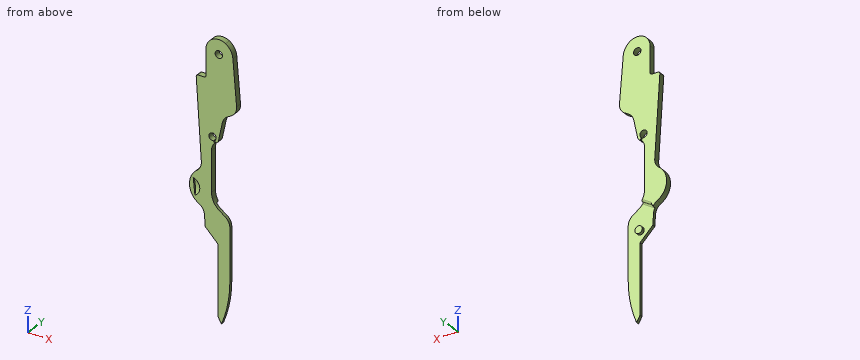
```python
from build123d import *

# Parameters (mm, degrees)
BOSS_EXTRUDE1_DEPTH     = 0.8
FILLET1_R               = 4.2
SKETCH2_R               = 1
CUT_EXTRUDE1_DEPTH      = 75.905340264
CUT_EXTRUDE2_DEPTH      = 75.905340264
CUT_EXTRUDE_THIN1_DEPTH = 75.905340264
FILLET2_R               = 3
CUT_EXTRUDE4_DEPTH      = 0.8
FILLET3_R               = 5
FILLET4_R               = 0.4
FILLET5_R               = 3
FILLET6_R               = 1
SKETCH6_R               = 1
BOSS_EXTRUDE2_DEPTH     = 0.8
SKETCH7_W               = 3
SKETCH7_H               = 11.1
CUT_EXTRUDE5_DEPTH      = 75.882809828
FILLET7_R               = 0.5
FILLET8_R               = 0.5
FILLET10_R              = 3.5
CUT_EXTRUDE6_DEPTH      = 0.5
FILLET11_R              = 2.4


# Some blends are built 0.0001 mm under size
with BuildPart() as part:
    # Sketch1 → Boss-Extrude1 (new, symmetric)
    with BuildSketch(Plane(origin=(0, 0, 0), x_dir=(1, 0, 0), z_dir=(0, 1, 0))):
        with BuildLine():
            Line((0, 0), (0, 6))
            Line((0, 6), (1.865312064, 35.32161706))
            ThreePointArc((1.865312064, 35.32161706), (-1.478238126, 40.437157563), (2.486591749, 45.087771133))
            Line((2.486591749, 45.087771133), (3.611473385, 62.770253978))
            ThreePointArc((3.611473385, 62.770253978), (4.720909281, 68.611088902), (7.232052008, 74))
            ThreePointArc((7.232052008, 74), (8.927699757, 68.307599169), (9.5, 62.395651864))
            Line((9.5, 62.395651864), (9.5, 46.645651864))
            Line((9.5, 46.645651864), (4.5, 43.144614173))
            Line((4.5, 43.144614173), (4.5, 27.994614173))
            Line((4.5, 27.994614173), (6.3, 26.955383689))
            Line((6.3, 26.955383689), (7.743698597, 20.163315799))
            Line((7.743698597, 20.163315799), (11.5, 17.994614173))
            Line((11.5, 17.994614173), (10, 0))
            Line((10, 0), (0, 0))
        make_face()
    extrude(amount=BOSS_EXTRUDE1_DEPTH, both=True)

    # Fillet1
    fillet1_edges = [part.edges().sort_by_distance(p)[0] for p in [
        (10, 0, 0),
    ]]
    fillet(fillet1_edges, radius=FILLET1_R)

    # Sketch2 → Cut-Extrude1 (cut, through all)
    with BuildSketch(Plane(origin=(0, 0.8, 0), x_dir=(1, 0, 0), z_dir=(0, 1, 0))):
        with Locations(Location((6.5, 4, 0), (0, 0, 270))):
            Circle(SKETCH2_R)
    extrude(amount=-CUT_EXTRUDE1_DEPTH, mode=Mode.SUBTRACT)

    # Sketch3 → Cut-Extrude2 (cut, through all)
    with BuildSketch(Plane(origin=(0, 0.8, 0), x_dir=(1, 0, 0), z_dir=(0, 1, 0))):
        with BuildLine():
            Line((5.640057539, 27.969251754), (5.047431638, 26.942793585))
            ThreePointArc((5.047431638, 26.942793585), (4.386066515, 25.063581102), (5.367538565, 26.797235046))
            Line((5.367538565, 26.797235046), (5.94316643, 27.794251754))
            Line((5.94316643, 27.794251754), (5.640057539, 27.969251754))
        make_face()
    extrude(amount=-CUT_EXTRUDE2_DEPTH, mode=Mode.SUBTRACT)

    # Sketch4 → Cut-Extrude-Thin1 (cut, through all)
    with BuildSketch(Plane(origin=(0, 0.8, 0), x_dir=(1, 0, 0), z_dir=(0, 1, 0))):
        Polygon((6.299086102, 72.375061168), (6.299086102, 53.5), (2.799086102, 50), (-4.271981709, 57.071067812), (-3.700913898, 57.642135624), (-3.700913898, 72.375061168), align=None)
    extrude(amount=-CUT_EXTRUDE_THIN1_DEPTH, mode=Mode.SUBTRACT)

    # Fillet2
    fillet2_edges = [part.edges().sort_by_distance(p)[0] for p in [
        (1.865312064, 0, -35.32161706),
        (2.486591749, 0, -45.087771133),
        (9.5, 0, -46.645651864),
    ]]
    fillet(fillet2_edges, radius=FILLET2_R)

    # Sketch5 → Cut-Extrude4 (cut)
    with BuildSketch(Plane(origin=(0, 0.8, 0), x_dir=(1, 0, 0), z_dir=(0, 1, 0))):
        Polygon((2.486591749, 45.087771133), (13.455116217, 38.22222401), (13.455116217, 80.886155846), (2.486591749, 80.886155846), (1.62289593, 47.027246142), align=None)
    extrude(amount=-CUT_EXTRUDE4_DEPTH, mode=Mode.SUBTRACT)

    # Fillet3
    fillet3_edges = [part.edges().sort_by_distance(p)[0] for p in [
        (4.5, 0, -43.144614173),
    ]]
    fillet(fillet3_edges, radius=FILLET3_R)

    # Fillet4
    fillet4_edges = [part.edges().sort_by_distance(p)[0] for p in [
        (3.91002639, 0, -44.196798274),
        (3.91002639, 0.8, -44.196798274),
    ]]
    fillet(fillet4_edges, radius=FILLET4_R - 0.0001)  # a hair under: the kernel refuses the full size

    # Fillet5
    # the kernel refuses this fillet: 3 mm, written as the material it adds along each edge
    with BuildSketch(Plane(origin=(4.5, 0.8, -27.994614173), x_dir=(0.8660254037844444, 0, 0.49999999999999023), z_dir=(0, -1, 0))) as fillet5_piece_1:
        with BuildLine():
            CenterArc((1.793781136, -2.893079935), FILLET5_R, 105.342812505, 44.657187495)
            Line((-0.804295075, -1.393079935), (0, 0))
            Line((0, 0), (1, 0))
        make_face()
    extrude(amount=1.6)
    with BuildSketch(Plane(origin=(7.743698597, 0.8, -20.163315799), x_dir=(0.8660254037844403, 0, 0.49999999999999734), z_dir=(0, -1, 0))) as fillet5_piece_2:
        with BuildLine():
            CenterArc((FILLET5_R * 0.445228685309, -FILLET5_R), FILLET5_R, 90, 48)
            Line((-FILLET5_R * 0.297916140169, -FILLET5_R * 0.330869393641), (0, 0))
            Line((0, 0), (FILLET5_R * 0.445228685309, 0))
        make_face()
    extrude(amount=1.6)
    # the kernel refuses this fillet: 3 mm, written as the material it takes off along each edge
    with BuildSketch(Plane(origin=(11.5, -5.55643762, -17.994614173), x_dir=(-0.86602540378444, 0, -0.49999999999999756), z_dir=(0, 1, 0))) as fillet5_2_piece_1:
        with BuildLine():
            CenterArc((FILLET5_R * 0.634191682642, FILLET5_R), FILLET5_R, 205.234939105, 64.765060895)
            Line((-FILLET5_R * 0.270375560362, FILLET5_R * 0.573669021903), (0, 0))
            Line((0, 0), (FILLET5_R * 0.634191682642, 0))
        make_face()
    extrude(amount=11.11287524, mode=Mode.SUBTRACT)

    # Fillet6
    fillet6_edges = [part.edges().sort_by_distance(p)[0] for p in [
        (6.3, 0, -26.955383689),
    ]]
    fillet(fillet6_edges, radius=FILLET6_R)

    # Sketch6 → Boss-Extrude2 (add)
    with BuildSketch(Plane(origin=(0, 0, 0), x_dir=(1, 0, 0), z_dir=(0, 1, 0))):
        with Locations(Location((6.14, 50.5, 0), (0, 0, 90))):
            Circle(SKETCH6_R)
    extrude(amount=BOSS_EXTRUDE2_DEPTH)

    # Sketch7 → Cut-Extrude5 (cut, through all)
    with BuildSketch(Plane(origin=(0, 0.8, 0), x_dir=(1, 0, 0), z_dir=(0, 1, 0))):
        with Locations((1.5, 5.55)):
            Rectangle(SKETCH7_W, SKETCH7_H)
    extrude(amount=-CUT_EXTRUDE5_DEPTH, mode=Mode.SUBTRACT)

    # Fillet7
    fillet7_edges = [part.edges().sort_by_distance(p)[0] for p in [
        (0.324439526, 0, -11.1),
    ]]
    fillet(fillet7_edges, radius=FILLET7_R)

    # Fillet8
    fillet8_edges = [part.edges().sort_by_distance(p)[0] for p in [
        (3, 0, -11.1),
    ]]
    fillet(fillet8_edges, radius=FILLET8_R)

    # Fillet10
    fillet10_edges = [part.edges().sort_by_distance(p)[0] for p in [
        (3, 0, 0),
    ]]
    fillet(fillet10_edges, radius=FILLET10_R)

    # Sketch8 → Cut-Extrude6 (cut)
    with BuildSketch(Plane.XZ.offset(0.8)):
        with BuildLine():
            Line((0, -42.705581243), (-0.472751816, -38.234175203))
            ThreePointArc((-0.472751816, -38.234175203), (1.308763911, -40.306514027), (0, -42.705581243))
        make_face()
    extrude(amount=-CUT_EXTRUDE6_DEPTH, mode=Mode.SUBTRACT)

    # Fillet11
    # the kernel refuses this fillet: 2.4 mm, written as the material it adds along each edge
    with BuildSketch(Plane(origin=(-1.081254443, -0.3, -40.559205352), x_dir=(-0.9553191525831795, 0, 0.2955762451682408), z_dir=(-0.2955762451682408, 0, -0.9553191525831795))) as fillet11_piece_1_section:
        with BuildLine():
            CenterArc((0.937051647, -2.4), FILLET11_R, 52.341537994, 37.658462006)
            Line((0.937051647, 0), (0.937051647, 0.048))
            Line((0.937051647, 0.048), (2.403339477, 0.048))
            Line((2.403339477, 0.048), (2.451339477, 0))
            ThreePointArc((2.451339477, 0), (2.451339477, -0.25), (2.432665233, -0.462))
            Line((2.432665233, -0.462), (2.403339477, -0.5))
        make_face()
    fillet11_piece_1 = revolve(axis=Axis((-1.081254443, -0.3, -40.559205352), (0, 1, 0)), revolution_arc=313.54514328, mode=Mode.PRIVATE)
    fillet11_piece_1 = split(fillet11_piece_1, bisect_by=Plane(origin=(-0.236375908, -0.3, -40.469878223), z_dir=(0.9944572448546122, 0, 0.1051417526778682)), keep=Keep.TOP, mode=Mode.PRIVATE)
    add(fillet11_piece_1)


solid = part.part
```
Build history of the part. All positions in model axes, mm. Round coordinates to 2 decimals unless told otherwise and drop trailing zeros. Write each loop counter-clockwise with the first axis right and the second up, starting at its lowest first coordinate (ties: lowest second). Pieces come first, ordered by that corner, then holes. Notation, with made-up numbers: (7.5, -40) - (16.5, -40) arc R28 ccw to (16.5, -8) - close; hole circle Ø1 at (88.25, -29.5). An arc over 180 degrees is marked (long way). Write each question's results on one line, items separated by ' | '. Start each with the question number.
Item 1: Saw through at A-A (z = -15). Write the cut outline in (x, y).
Item 2: Saw through at B-B (z = -37). Write the cut outline in (x, y), and give its area (3 significant figures).
Item 3: Wall check: L1, parallel to X at y = 0.55, z = -4; L2, parallel to Y at x = 5.25, z = -44; L3, parallel to Z at x = 6, y = 0.25. Give the ranges that are in metal, low to high. Write a range as [from, to].
Item 4: Drop flat-ended pins along their axis: P1, Ø6, axis at x = 7, z = -66.5, coming from the +Y side; P2, Ø0.9, axis at y = -0.5, z = -59, coming from the -X side; P3, Ø0.5, axis at y = 0.5, z = -6.5, coming from the -X side. Give the stop position or say it passes through.
Results are:
1) outline: (0.57, -0.8) - (11.25, -0.8) - (11.25, 0.8) - (0.57, 0.8) - close
2) outline: (-0.43, -0.8) - (4.5, -0.8) - (4.5, 0.8) - (-0.43, 0.8) - close | area: 7.88 mm²
3) L1: x = [3, 5.5], [7.5, 10.33] | L2: y = [-0.8, 0] | L3: z = [-51.49, -49.51], [-27.12, -4.87], [-3.13, -0.14]
4) P1: stops at y = 0 | P2: stops at x = 6.3 | P3: stops at x = 3
